```python
from build123d import *

# Parameters (mm, degrees)
F0_W     = 109.774076
F0_H     = 77.548884
F1_DEPTH = 63.5
F2_W     = 96.05325
F2_H     = 52.179004
F3_DEPTH = 63.5
F4_W     = 81.802986
F4_H     = 63.615836
F5_DEPTH = 63.5
F6_W     = 47.944924
F6_H     = 38.00063
F7_DEPTH = 101.6
F8_R     = 6.312248
F9_DEPTH = 254


with BuildPart() as f1:
    # F0 (on Top) → F1 (new body)
    with BuildSketch(Plane.XY):
        Rectangle(F0_W, F0_H)
    extrude(amount=F1_DEPTH)

    # F2 (on Top) → F3 (cut)
    with BuildSketch(Plane.XY):
        Rectangle(F2_W, F2_H)
    extrude(amount=F3_DEPTH, mode=Mode.SUBTRACT)

    # F4 (on Top) → F5 (cut)
    with BuildSketch(Plane.XY):
        Rectangle(F4_W, F4_H)
    extrude(amount=-F5_DEPTH, mode=Mode.SUBTRACT)

    # F6 (on face) → F7 (cut)
    with BuildSketch(Plane.XZ.offset(38.774442)):
        with Locations((-0.610764, 44.499685)):
            Rectangle(F6_W, F6_H)
    extrude(amount=-F7_DEPTH, mode=Mode.SUBTRACT)

    # F8 (on face) → F9 (cut)
    with BuildSketch(Plane.YZ.offset(54.887038)):
        with Locations((0, 13.589485)):
            Circle(F8_R)
    extrude(amount=-F9_DEPTH, mode=Mode.SUBTRACT)


solid = f1.part
```
Input: part model. Units: mm. Frame: model coordinates. A direction names the side the tool comes from. Coordinates: 2 decimals unless noted, no trailing zeros. Loops run counter-clockwise (first coordinate to the right, second up) from the corner with the lowest first, then second, coordinate; pieces in that order, holes last. Notation, with made-up numbers: M 66.5,38 L 80.5,38 A13 cw 80.5,60 Z; hole C 72,-22.5 d11. An arc over 180 degrees is marked long. Answer in a Markdown table with one row per item.
1. Section D-D, the plane y = 0. Output: boundary loops of the cut face in (x, z).
Response:
| item | result |
|---|---|
| outline | M -54.89,0 L -48.03,0 L -48.03,7.28 L -54.89,7.28 Z; M -54.89,19.9 L -48.03,19.9 L -48.03,63.5 L -54.89,63.5 Z; M 48.03,0 L 54.89,0 L 54.89,7.28 L 48.03,7.28 Z; M 48.03,19.9 L 54.89,19.9 L 54.89,63.5 L 48.03,63.5 Z |
2. Draft query along Y for faces 4 (the flat face through (-54.887, -1, 31)), 5 (the flat face through (-48.027, 0, 31)), 6 (the flat face through (-1, 38.774, 24)). Return one class per face: pulls with the +Y half, pulls with the -Y half, needs draft (parallel to the pull), parting line crosses it, or undercut.
Response:
| item | result |
|---|---|
| face 4 | needs draft |
| face 5 | undercut |
| face 6 | pulls with the +Y half |
3. First-contact query: pin 1 (4 mm diameter, centred on x = -5, y = 34, fed in from +Z). Flat tip, straight axial feed; report the tip coordinate or a pass-through.
Response:
| item | result |
|---|---|
| pin 1 | stops at z = 25.5 |
4. Section C-C, the plane y = 16. Output: boundary loops of the cut face in (x, z), then the cut area to 3 significant figures.
Response:
| item | result |
|---|---|
| outline | M -54.89,0 L -48.03,0 L -48.03,63.5 L -54.89,63.5 Z; M 48.03,0 L 54.89,0 L 54.89,63.5 L 48.03,63.5 Z |
| area | 871 mm2 |
5. Reachability of faces 1 (the flat face through (-24.583, -33, 44)), 2 (the flat face through (-13, 26.4, 0)), 3 (the flat face through (-1, 26.09, 24)) from +Z, -Z, +X, -X, +Y, -Y: full face, straight path, thin tool, end or side. Return the list, or none.
Response:
| item | result |
|---|---|
| face 1 | +Z, +Y, -Y |
| face 2 | -Z, +X, -X, +Y, -Y |
| face 3 | +Z, -Z |
6. Material intervals for line 1 (Y direction, x = 46.5, z = 56); line 2 (Z direction, x = -52, y = 0); line 3 (X direction, y = -28.5, z = 56), sorted ascending.
Response:
| item | result |
|---|---|
| line 1 | y = -38.77 to -26.09, 26.09 to 38.77 |
| line 2 | z = 0 to 7.28, 19.9 to 63.5 |
| line 3 | x = -54.89 to -24.58, 23.36 to 54.89 |
7. Section B-B, the plane z = 59.5. Output: boundary loops of the cut face in (x, y), then the cut area to 3 significant figures.
Response:
| item | result |
|---|---|
| outline | M -54.89,-38.77 L -24.58,-38.77 L -24.58,-26.09 L -48.03,-26.09 L -48.03,26.09 L -24.58,26.09 L -24.58,38.77 L -54.89,38.77 Z; M 23.36,-38.77 L 54.89,-38.77 L 54.89,38.77 L 23.36,38.77 L 23.36,26.09 L 48.03,26.09 L 48.03,-26.09 L 23.36,-26.09 Z |
| area | 2,280 mm2 |
8. Section A-A, the plane x = 5.5. Output: boundary loops of the cut face in (y, z), then the cut area to 3 significant figures.
Response:
| item | result |
|---|---|
| outline | M -38.77,0 L -26.09,0 L -26.09,25.5 L -38.77,25.5 Z; M 26.09,0 L 38.77,0 L 38.77,25.5 L 26.09,25.5 Z |
| area | 647 mm2 |
